Model file for the job. Use its own axes, mm. Face numbers are marked on the shaded views. A direction names the side the tool comes from. Coordinates: 2 decimals unless noted, no trailing zeros. Write each loop counter-clockwise with the first axis right and the second up, starting at its lowest first coordinate (ties: lowest second). Pieces come first, ordered by that corner, then holes.
Q1. Band-saw the part on B-B, the plane x = 0. Write the cut outline in (y, z) (3 decimals), plus the area to 3 significant figures.
Q2. Drill centre lines: probe 1 along Z at (x, y) = (-4.5, 0); probe 2 along Y at (x, z) = (0, 6.5); probe 3 along Z at (x, y) = (0, 11). Where is each one in solid material? Low to high.
Q3. Band-saw the part on C-C, the plane z = 3. Write the cut outline in (x, y), plus the area to 3 significant figures.
Q4. Pull direction X, two halves, no side cores. Call the marked faces 1, 2 and 3: released by +X, released by -X, zero draft, split by the parting line, or undercut.
Q5. Pin check, flat tips, straight feed: P1, Ø1.5, axis at y = 6, z = 8.5, coming from the +X side; P2, Ø5, axis at x = -2, z = 10, coming from the -Y side; P3, Ø1.5, axis at x = 12, y = 5.5, coming from the +Z side. Stop position of each tip, or through.
Q6. Which spindle directions (+Z, -Z, +X, -X, +Y, -Y) get a long thin tool onto all of the face, cutting with end or side? Do the marked faces 4 and 5. Say none if no direction does.
Q7. Band-saw the part on A-A, the plane y = 0. Write the cut outline in (x, z) (3 decimals), plus the area to 3 significant figures.
from build123d import *

# Parameters (mm, degrees)
F0_R     = 19.05
F1_DEPTH = 7.62
F2_R     = 9.525
F3_DEPTH = 6.35
F4_R     = 1.905
F5_DEPTH = 25.4
F6_R     = 2.286
F7_DEPTH = 101.6
F8_R     = 1.27


with BuildPart() as f1:
    # F0 (on Top) → F1 (new body)
    with BuildSketch(Plane.XY):
        Circle(F0_R)
    extrude(amount=F1_DEPTH)

    # F2 (on face) → F3 (join)
    with BuildSketch(Plane.XY.offset(7.62)):
        Circle(F2_R)
    extrude(amount=F3_DEPTH)

    # F4 (on Right) → F5 (cut)
    with BuildSketch(Plane.YZ):
        with Locations((0, 10.795)):
            Circle(F4_R)
    extrude(amount=-F5_DEPTH, mode=Mode.SUBTRACT)

    # F6 (on face) → F7 (cut)
    with BuildSketch(Plane(origin=(0, 0, 0), x_dir=(1, 0, 0), z_dir=(0, 0, -1))):
        Circle(F6_R)
    extrude(amount=-F7_DEPTH, mode=Mode.SUBTRACT)

    # F8 (on Right) → F9 (revolve, cut)
    with BuildSketch(Plane.YZ):
        with Locations((-19.05, 3.81)):
            Circle(F8_R)
    revolve(axis=Axis((0, 0, 13.97), (0, 0, 1)), mode=Mode.SUBTRACT)


solid = f1.part
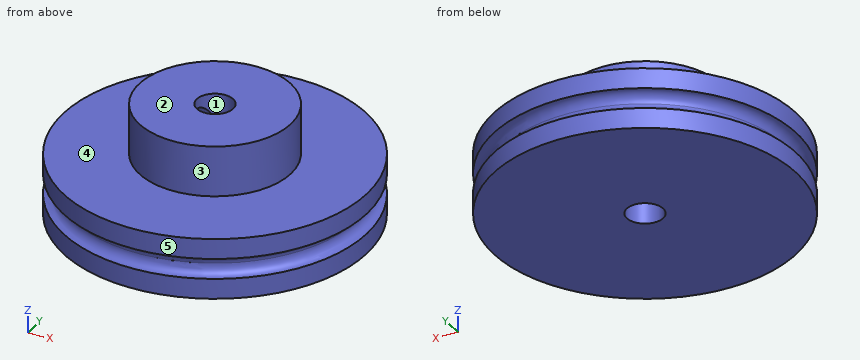
Answer sheet:
1. outline: (-19.05, 0) - (-2.286, 0) - (-2.286, 13.97) - (-9.525, 13.97) - (-9.525, 7.62) - (-19.05, 7.62) - (-19.05, 5.08) arc R1.27 cw to (-19.05, 2.54) - close; (2.286, 0) - (19.05, 0) - (19.05, 2.54) arc R1.27 cw to (19.05, 5.08) - (19.05, 7.62) - (9.525, 7.62) - (9.525, 13.97) - (2.286, 13.97) - close
1. area: 342 mm2
2. probe 1: z = 0 to 8.89, 12.7 to 13.97
2. probe 2: y = -19.05 to -2.29, 2.29 to 19.05
2. probe 3: z = 0 to 7.62
3. outline: circle Ø36.14 at (0, 0); hole circle Ø4.57 at (0, 0)
3. area: 1,010 mm2
4. face 1: undercut
4. face 2: zero draft
4. face 3: split by the parting line
5. P1: stops at x = 7.95
5. P2: stops at y = -19.01
5. P3: stops at z = 7.62
6. face 4: +Z
6. face 5: +Z, -Z
7. outline: (-19.05, 0) - (-2.286, 0) - (-2.286, 8.89) - (-9.525, 8.89) - (-9.525, 7.62) - (-19.05, 7.62) - (-19.05, 5.08) arc R1.27 cw to (-19.05, 2.54) - close; (-9.525, 12.7) - (-2.286, 12.7) - (-2.286, 13.97) - (-9.525, 13.97) - close; (2.286, 0) - (19.05, 0) - (19.05, 2.54) arc R1.27 cw to (19.05, 5.08) - (19.05, 7.62) - (9.525, 7.62) - (9.525, 13.97) - (2.286, 13.97) - close
7. area: 315 mm2
